Input: part model. Units: mm. Frame: model coordinates. Round coordinates to 2 decimals unless told otherwise and drop trailing zeros. Loops run counter-clockwise (first coordinate to the right, second up) from the corner with the lowest first, then second, coordinate; pieces in that order, holes last. Notation, with made-up numbers: (-27.75, -4) - (-17.75, -4) arc R8 ccw to (-17.75, 9) - close; hole circle Ø5 at (81.5, 44). An arc over 180 degrees is marked (long way). One line per question, with ' | ' between items. Start each with the question number.
Item 1: Section A-A, the plane z = -82.55. Return loops of the section in (x, y) (3 decimals), plus the area to 3 significant figures.
Item 2: Section C-C, the plane z = -38. Return loops of the section in (x, y).
Item 3: Section B-B, the plane z = -20.5. Return loops of the section in (x, y).
Item 4: Material intervals for line 1 along X through (y, z) = (1.85, -82.55); line 2 along Z through (x, y) = (11, 2.5) (3 decimals); line 3 along X through (y, z) = (1.5, -48), sorted ascending.
Item 5: First-contact query: pin 1 (3 mm diameter, centred on x = 50.5, y = 3.5, fed in from -Z); pin 2 (1.9 mm diameter, centred on y = 4.5, z = 2, fed in from -X); pin 3 (1.4 mm diameter, centred on x = 54.14, z = -82.55, fed in from -Y); pin 4 (1.6 mm diameter, centred on x = 53.5, z = -82, fed in from +Y) (3 decimals). Flat tips, straight axial feed; report the tip coordinate or a pass-through.
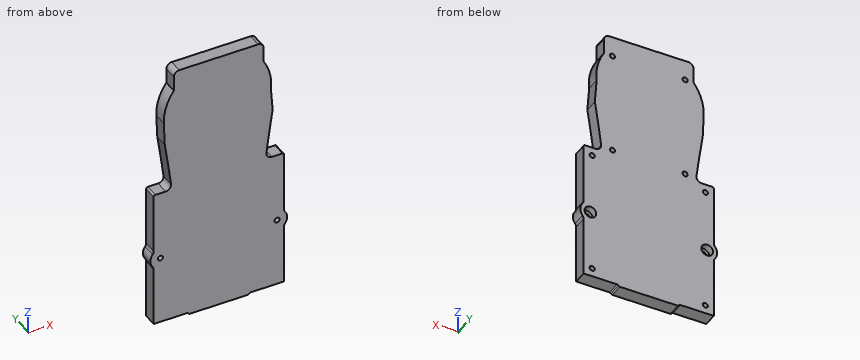
```python
from build123d import *

# Parameters (mm, degrees)
SKETCH1_R           = 1.190625
BOSS_EXTRUDE1_DEPTH = 6.35
SKETCH2_R           = 1.190625
CUT_EXTRUDE1_DEPTH  = 5.953125
SKETCH3_R           = 2.728515752
CUT_EXTRUDE2_DEPTH  = 3.175


with BuildPart() as part:
    # Sketch1 → Boss-Extrude1 (new body)
    with BuildSketch(Plane(origin=(0, 0, 0), x_dir=(1, 0, 0), z_dir=(0, 1, 0))):
        with BuildLine():
            ThreePointArc((57.271558663, 87.137426409), (57.399480252, 86.341513261), (57.770360032, 85.625768991))
            ThreePointArc((57.770360032, 85.625768991), (58.78527106, 82.55), (57.770360032, 79.474231009))
            ThreePointArc((57.770360032, 79.474231009), (57.399480252, 78.758486739), (57.271558663, 77.962573591))
            Line((57.271558663, 77.962573591), (57.271558663, 50.187158197))
            ThreePointArc((57.271558663, 50.187158197), (57.006550783, 49.778004586), (56.529846621, 49.676078162))
            Line((56.529846621, 49.676078162), (52.561739328, 49.676078162))
            Line((52.561739328, 49.676078162), (51.683486492, 49.676078162))
            ThreePointArc((51.683486492, 49.676078162), (49.779800182, 48.817618657), (49.162915139, 46.822517874))
            ThreePointArc((49.162915139, 46.822517874), (50.534142833, 36.419600029), (52.056928392, 26.037784715))
            Line((52.056928392, 26.037784715), (51.254736023, 14.952744828))
            ThreePointArc((51.254736023, 14.952744828), (50.812383961, 7.190984278), (47.857667851, 0))
            Line((47.857667851, 0), (47.857667851, -6.985))
            ThreePointArc((47.857667851, -6.985), (47.113719075, -8.781051224), (45.317667851, -9.525))
            Line((45.317667851, -9.525), (8.657332149, -9.525))
            ThreePointArc((8.657332149, -9.525), (6.861280925, -8.781051224), (6.117332149, -6.985))
            Line((6.117332149, -6.985), (6.117332149, 0))
            ThreePointArc((6.117332149, 0), (2.495961134, 7.074805948), (1.444635194, 14.952744828))
            Line((1.444635194, 14.952744828), (1.918071608, 26.037784715))
            ThreePointArc((1.918071608, 26.037784715), (3.440857167, 36.419600029), (4.812084861, 46.822517874))
            ThreePointArc((4.812084861, 46.822517874), (4.195199818, 48.817618657), (2.291513508, 49.676078162))
            Line((2.291513508, 49.676078162), (-2.470986492, 49.676078162))
            ThreePointArc((-2.470986492, 49.676078162), (-3.032252499, 49.908562155), (-3.264736492, 50.469828162))
            Line((-3.264736492, 50.469828162), (-3.264736492, 77.962573591))
            ThreePointArc((-3.264736492, 77.962573591), (-3.392658081, 78.758486739), (-3.763537861, 79.474231009))
            ThreePointArc((-3.763537861, 79.474231009), (-4.778448889, 82.55), (-3.763537861, 85.625768991))
            ThreePointArc((-3.763537861, 85.625768991), (-3.392658081, 86.341513261), (-3.264736492, 87.137426409))
            Line((-3.264736492, 87.137426409), (-3.264736492, 114.763578162))
            Line((-3.264736492, 114.763578162), (12.197441337, 114.763578162))
            ThreePointArc((12.197441337, 114.763578162), (12.594316337, 114.869920498), (12.884849002, 115.160453162))
            ThreePointArc((12.884849002, 115.160453162), (13.175381666, 115.450985826), (13.572256666, 115.557328162))
            Line((13.572256666, 115.557328162), (40.402743334, 115.557328162))
            ThreePointArc((40.402743334, 115.557328162), (40.799618334, 115.450985826), (41.090150998, 115.160453162))
            ThreePointArc((41.090150998, 115.160453162), (41.380683663, 114.869920498), (41.777558663, 114.763578162))
            Line((41.777558663, 114.763578162), (57.271558663, 114.763578162))
            Line((57.271558663, 114.763578162), (57.271558663, 87.137426409))
        make_face()
        with Locations((54.141854512, 82.55)):
            Circle(SKETCH1_R, mode=Mode.SUBTRACT)
        with Locations((-0.166854512, 82.55)):
            Circle(SKETCH1_R, mode=Mode.SUBTRACT)
    extrude(amount=BOSS_EXTRUDE1_DEPTH)

    # Sketch2 → Cut-Extrude1 (cut)
    with BuildSketch(Plane(origin=(0, 6.35, 0), x_dir=(1, 0, 0), z_dir=(0, 1, 0))):
        with Locations((10.086082149, 0)):
            Circle(SKETCH2_R)
        with Locations((43.888917851, 0)):
            Circle(SKETCH2_R)
        with Locations((10.086082149, 47.625)):
            Circle(SKETCH2_R)
        with Locations((43.888917851, 47.625)):
            Circle(SKETCH2_R)
        with Locations((0.704013508, 53.644828162)):
            Circle(SKETCH2_R)
        with Locations((0.704013508, 110.794828162)):
            Circle(SKETCH2_R)
        with Locations((53.302808663, 53.644828162)):
            Circle(SKETCH2_R)
        with Locations((53.302808663, 110.794828162)):
            Circle(SKETCH2_R)
    extrude(amount=-CUT_EXTRUDE1_DEPTH, mode=Mode.SUBTRACT)

    # Sketch3 → Cut-Extrude2 (cut)
    with BuildSketch(Plane(origin=(0, 6.35, 0), x_dir=(1, 0, 0), z_dir=(0, 1, 0))):
        with Locations((-0.166854512, 82.55)):
            Circle(SKETCH3_R)
        with Locations((54.141854512, 82.55)):
            Circle(SKETCH3_R)
    extrude(amount=-CUT_EXTRUDE2_DEPTH, mode=Mode.SUBTRACT)


solid = part.part
```
Return value:
1) outline: (-4.778, 0) - (-1.357, 0) - (-1.357, 3.175) - (-2.895, 3.175) - (-2.895, 6.35) - (-4.778, 6.35) - close; (1.024, 0) - (52.951, 0) - (52.951, 3.175) - (51.413, 3.175) - (51.413, 6.35) - (2.562, 6.35) - (2.562, 3.175) - (1.024, 3.175) - close; (55.332, 0) - (58.785, 0) - (58.785, 6.35) - (56.87, 6.35) - (56.87, 3.175) - (55.332, 3.175) - close | area: 354 mm2
2) outline: (3.66, 0) - (50.32, 0) - (50.32, 6.35) - (3.66, 6.35) - close
3) outline: (1.68, 0) - (51.66, 0) - (51.66, 6.35) - (1.68, 6.35) - close
4) line 1: -4.78 to -1.36, 1.02 to 52.95, 55.33 to 58.79 | line 2: -114.764 to -48.388, -46.862 to -0.763, 0.763 to 9.525 | line 3: 4.68 to 8.96, 11.22 to 42.76, 45.02 to 49.29
5) pin 1: z = -114.76 | pin 2: x = 6.12 | pin 3: through | pin 4: y = 3.175
